from build123d import *

# Parameters (mm, degrees)
F0_W     = 40
F0_H     = 90
F1_DEPTH = 8
F2_W     = 40
F2_H     = 15
F3_DEPTH = 30
F4_W     = 40
F4_H     = 10
F5_DEPTH = 30
F6_R     = 7.99999
F7_SIZE2 = 10
F7_SIZE  = 10


# Not quite as in the source:
# - a fillet or chamfer is up to 0.001 mm smaller than in the source, because OpenCascade refuses the exact size


with BuildPart() as f1:
    # F0 (on Top) → F1 (new body)
    with BuildSketch(Plane.XY):
        with Locations((-20, 7.0996452868)):
            Rectangle(F0_W, F0_H)
    extrude(amount=F1_DEPTH)

    # F2 (on face) → F3 (join)
    with BuildSketch(Plane(origin=(0, 0, 0), x_dir=(1, 0, 0), z_dir=(0, 0, -1))):
        with Locations((-20, 5.4003547132)):
            Rectangle(F2_W, F2_H)
    extrude(amount=F3_DEPTH)

    # F4 (on face) → F5 (join)
    with BuildSketch(Plane(origin=(0, 2.0996452868, 0), x_dir=(-1, 0, 0), z_dir=(0, 1, 0))):
        with Locations((20, -25)):
            Rectangle(F4_W, F4_H)
    extrude(amount=F5_DEPTH)

    # F6 (radius 8 in the source; OpenCascade refuses exactly that, so slightly less here)
    f6_edges = [f1.edges().sort_by_distance(p)[0] for p in [
        (0, 7.099645, 8),
        (-40, 7.099645, 8),
    ]]
    fillet(f6_edges, radius=F6_R)

    # F7
    f7_edges = [f1.edges().sort_by_distance(p)[0] for p in [
        (-20, -12.900355, -30),
    ]]
    chamfer(f7_edges, length=F7_SIZE, length2=F7_SIZE2)


solid = f1.part
Work out the finished part from the listing and answer in its coordinate system (mm). A direction names the side the tool comes from. Give positions to 0.01 mm unless a question says otherwise; leave off trailing zeros. Order: outer loops, then holes, each group sorted by start corner. A loop starts at its lowest first (then second) coordinate and runs counter-clockwise, first axis right, second up. Notation, with made-up numbers: (75.25, -1) - (98.25, -1) arc R28 cw to (98.25, 29) - close; hole circle Ø5 at (36.25, 65). An arc over 180 degrees is marked (long way). Answer as CSV lines item,"result". Start each with the question number.
Q1. The mould has two halves that part along Z. Classify faces 6 (the face through (-20, 52.1, 4)), 7 (the face through (-20.3, -7.8, -25.1)), 8 (the face through (-20, 27, 0)): +Z half, -Z half, draft (parallel to the pull), parting line (faces both ways), or undercut.
Q2. For faces 1 (the face through (-20, 17, -20)), 2 (the face through (-20, -37.9, 4)), 3 (the face through (-37.719, 7.73, 5.594)), 4 (the face through (-20, 32.1, -25)), 5 (the face through (-20, -12.9, -10)), determine the directions among +Z, -Z, +X, -X, +Y, -Y from which every point of the face is accessible in a straight line to the end or side of a thin tool.
Q3. Find the intervals of material crossed by L1, parallel to Z at x = -27.5, y = 17; L2, parallel to Z at x = -9.5, y = -16; L3, parallel to Y at x = -4, z = -7.5, in increasing order. Write a range as [from, to].
Q4. The part is cut by section D-D (z = -1). Write down the section's boundary in (x, y).
Q5. Given pin 1 Ø6 at (x, z) = (-16.5, -7.5) entering from -Y; pin 2 Ø10 at (x, z) = (-22, -10) entering from +Y; pin 3 Ø10 at (x, y) = (-20.5, 35) entering from -Z; pin 4 Ø20 at (x, y) = (-29.5, -27) entering from -Z, each flat-ended and moving along its own axis, determine where each tip first touches the part or whether it passes through.
Q6. The part is cut by section B-B (x = -18). Write down the section's boundary in (y, z).
Check result:
1,face 6,"draft"
1,face 7,"-Z half"
1,face 8,"undercut"
2,face 1,"+X, -X, +Y"
2,face 2,"+Z, -Z, +X, -X, -Y"
2,face 3,"+Z, -X, +Y, -Y"
2,face 4,"-Z, +X, -X, +Y"
2,face 5,"-Z, +X, -X, -Y"
3,L1,"z = [-30, -20], [0, 8]"
3,L2,"z = [0, 8]"
3,L3,"y = [-12.9, 2.1]"
4,outline,"(-40, -12.9) - (0, -12.9) - (0, 2.1) - (-40, 2.1) - close"
5,pin 1,"stops at y = -12.9"
5,pin 2,"stops at y = 2.1"
5,pin 3,"stops at z = -30"
5,pin 4,"stops at z = 0"
6,outline,"(-37.9, 0) - (-12.9, 0) - (-12.9, -20) - (-2.9, -30) - (32.1, -30) - (32.1, -20) - (2.1, -20) - (2.1, 0) - (52.1, 0) - (52.1, 8) - (-37.9, 8) - close"
